Could you check a few things on this drawing? It's one solid part, dimensions in mm from its lowest x, y, z. A direction names the side the tool comes from. Give positions to 0.01 mm unless a question says otherwise; leave off trailing zeros. Loops run counter-clockwise (first coordinate to the right, second up) from the corner with the lowest first, then second, coordinate; pieces in that order, holes last. Notation, with made-up numbers: M 27,70.25 L 33,70.25 A32 cw 33,100.25 Z; hole C 18,49 d9. An arc over 180 degrees is marked long. Answer in a Markdown table with one row per item. Add a question column.
1. If we section it at B-B on y = 49: List the corners of the cut face in (x, z) for me, then the cut area to 3 significant figures.
2. Thinking about a two-plate mould opening in X: for the marked faces 1, 2 and 3, which applies, released by +X, released by -X, zero draft, split by the parting line, or undercut?
3. If we section it at A-A on z = 43.5: List the corners of the cut face in (x, y) for me, then the cut area to 3 significant figures.
4. Which directions (+Z, -Z, +X, -X, +Y, -Y) give clear straight access to the entire face, cutting with the end or side of a thin tool? Please do the marked faces 4, 5 and 6.
5. If we section it at C-C on z = 55.5: List the corners of the cut face in (x, y) for me.
6. If we section it at D-D on y = 55.5: List the corners of the cut face in (x, z) for me.
7. I'm going to push flat-ended pins straight in: pin 1 Ø12 at (x, y) = (39, 43.5) entering from -Z; pin 2 Ø9.5 at (x, z) = (31.5, 8.5) entering from +Y; pin 3 Ø1.9 at (y, z) = (45.5, 59) entering from -X. Where does each tip first touch, or does it pass through?
8. I need wall thicknesses on line 1 along Y through (x, z) = (10, 55); line 2 along Y through (x, z) = (16, 4.5); line 3 along Y through (x, z) = (59, 56.5). Which ranges of each line are inside material? Lowest first, please. Write a range as from..to.
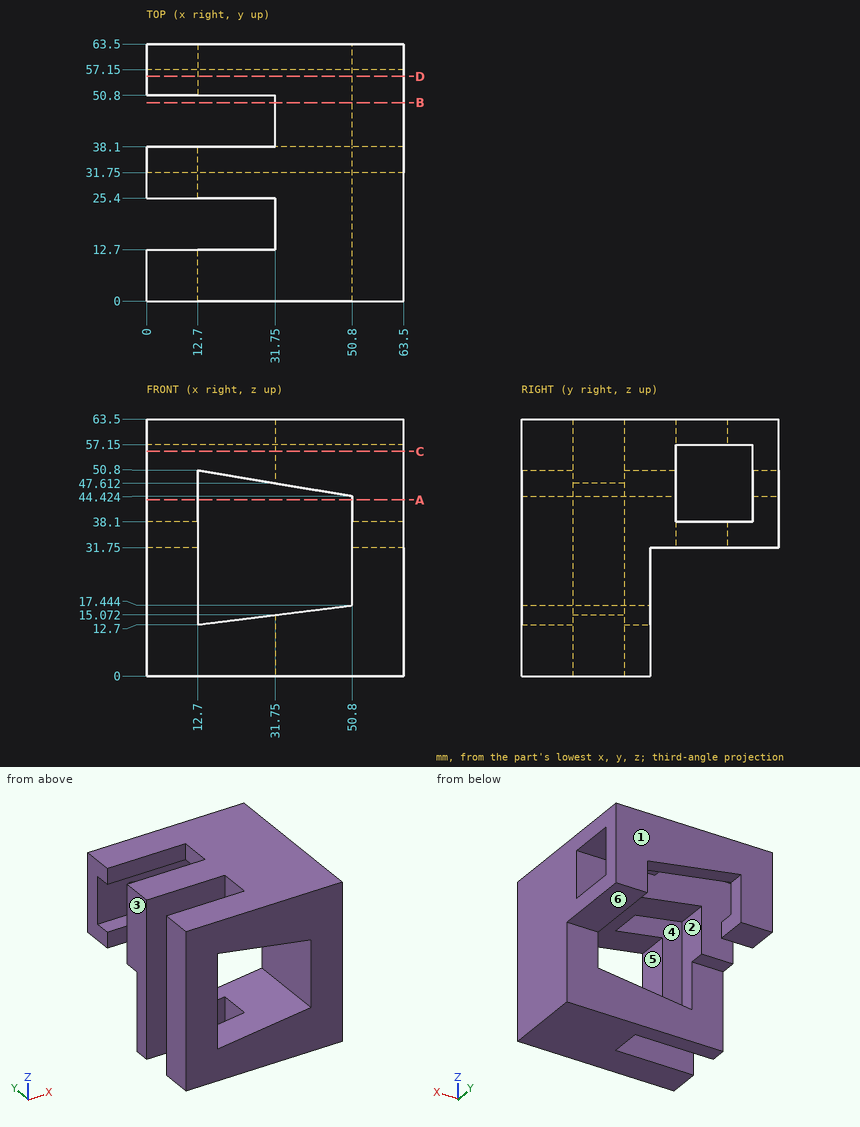
Results:
| question | item | result |
|---|---|---|
| 1 | outline | M 31.75,57.15 L 63.5,57.15 L 63.5,63.5 L 31.75,63.5 Z; M 50.8,31.75 L 63.5,31.75 L 63.5,38.1 L 50.8,38.1 Z |
| 1 | area | 282 mm2 |
| 2 | face 1 | zero draft |
| 2 | face 2 | undercut |
| 2 | face 3 | released by -X |
| 3 | outline | M 0,0 L 12.7,0 L 12.7,12.7 L 0,12.7 Z; M 0,25.4 L 12.7,25.4 L 12.7,38.1 L 0,38.1 Z; M 0,57.15 L 12.7,57.15 L 12.7,63.5 L 0,63.5 Z; M 50.8,0 L 63.5,0 L 63.5,38.1 L 50.8,38.1 Z; M 50.8,57.15 L 63.5,57.15 L 63.5,63.5 L 50.8,63.5 Z |
| 3 | area | 968 mm2 |
| 4 | face 4 | +Z, -Z, -X |
| 4 | face 5 | +Y, -Y |
| 4 | face 6 | -Z, +X, -X, +Y |
| 5 | outline | M 0,0 L 63.5,0 L 63.5,38.1 L 0,38.1 L 0,25.4 L 31.75,25.4 L 31.75,12.7 L 0,12.7 Z; M 0,57.15 L 63.5,57.15 L 63.5,63.5 L 0,63.5 Z |
| 6 | outline | M 0,31.75 L 12.7,31.75 L 12.7,38.1 L 0,38.1 Z; M 0,57.15 L 63.5,57.15 L 63.5,63.5 L 0,63.5 Z; M 50.8,31.75 L 63.5,31.75 L 63.5,38.1 L 50.8,38.1 Z |
| 7 | pin 1 | z = 45.96 |
| 7 | pin 2 | y = 31.75 |
| 7 | pin 3 | x = 31.75 |
| 8 | line 1 | 0..12.7, 25.4..38.1, 57.15..63.5 |
| 8 | line 2 | 0..12.7, 25.4..31.75 |
| 8 | line 3 | 0..38.1, 57.15..63.5 |
